Read the model definition and answer for the solid it produces. Units are mm, in the model's axes. Round coordinates to 2 decimals unless told otherwise and drop trailing zeros. Order: outer loops, then holes, each group sorted by start corner. A loop starts at its lowest first (then second) coordinate and runs counter-clockwise, first axis right, second up. Notation, with made-up numbers: (84.5, -8.75) - (90.5, -8.75) arc R26 cw to (90.5, 26.25) - close; hole circle Ø2 at (41.5, 60). An arc over 180 degrees is marked (long way). Answer as a JSON object with one key per item and string values. Group by question number.
Q1. Given pin 1 Ø2.5 at (y, z) = (-2, 1.5) entering from +X; pin 2 Ø1.5 at (x, y) = (-26, -2.5) entering from -Z; pin 3 Ø1 at (x, y) = (-6, -2.5) entering from -Z, each flat-ended and moving along its own axis, determine where each tip first touches the part or whether it passes through.
Q2. A cutting plane is placed at D-D on z = 83.5. Determine the outline of the cut face in (x, y), and give its area (3 significant figures).
Q3. A cutting plane is placed at C-C on y = -3.8. Count the separate pieces of the cut face and the enclosed holes in it, and give its area (3 significant figures).
Q4. A cutting plane is placed at A-A on z = -22. Determine the outline of the cut face in (x, y).
Q5. Consider line 1 (Z direction, x = 52.5, y = -4.3); line 2 (X direction, y = -3.75, z = 48); line 3 (X direction, y = -4, z = 62). Determine where each line is inside the solid, lowest interval first.
Q6. A cutting plane is placed at B-B on z = 108.5. Determine the outline of the cut face in (x, y), and give its area (3 significant figures).
```python
from build123d import *

# Parameters (mm, degrees)
SKETCH2_R           = 2.5
SKETCH2_W           = 5
SKETCH2_H           = 60
BOSS_EXTRUDE1_DEPTH = 5
BOSS_EXTRUDE2_DEPTH = 5


with BuildPart() as part:
    # Sketch2 → Boss-Extrude1 (new body)
    with BuildSketch(Plane(origin=(0, 0, 0), x_dir=(1, 0, 0), z_dir=(0, 1, 0))):
        with BuildLine():
            Line((45, 75), (75, 45))
            ThreePointArc((75, 45), (56.360389693, 0), (75, -45))
            Line((75, -45), (45, -75))
            ThreePointArc((45, -75), (0, -56.360389693), (-45, -75))
            Line((-45, -75), (-75, -45))
            ThreePointArc((-75, -45), (-56.360389693, 0), (-75, 45))
            Line((-75, 45), (-45, 75))
            ThreePointArc((-45, 75), (0, 56.360389693), (45, 75))
        make_face()
        with Locations(Location((50.841633347, 30.621504688, 0), (0, 0, 270))):
            Circle(SKETCH2_R, mode=Mode.SUBTRACT)
        with Locations(Location((61.448235065, 41.228106405, 0), (0, 0, 270))):
            Circle(SKETCH2_R, mode=Mode.SUBTRACT)
        with Locations(Location((30.621504688, 50.841633347, 0), (0, 0, 90))):
            Circle(SKETCH2_R, mode=Mode.SUBTRACT)
        with Locations(Location((41.228106405, 61.448235065, 0), (0, 0, 90))):
            Circle(SKETCH2_R, mode=Mode.SUBTRACT)
        with Locations(Location((30.621504688, -50.841633347, 0), (0, 0, 270))):
            Circle(SKETCH2_R, mode=Mode.SUBTRACT)
        with Locations(Location((41.228106405, -61.448235065, 0), (0, 0, 270))):
            Circle(SKETCH2_R, mode=Mode.SUBTRACT)
        with Locations(Location((61.448235065, -41.228106405, 0), (0, 0, 90))):
            Circle(SKETCH2_R, mode=Mode.SUBTRACT)
        with Locations(Location((50.841633347, -30.621504688, 0), (0, 0, 90))):
            Circle(SKETCH2_R, mode=Mode.SUBTRACT)
        with Locations(Location((-50.841633347, -30.621504688, 0), (0, 0, 270))):
            Circle(SKETCH2_R, mode=Mode.SUBTRACT)
        with Locations(Location((-61.448235065, -41.228106405, 0), (0, 0, 270))):
            Circle(SKETCH2_R, mode=Mode.SUBTRACT)
        with Locations(Location((-41.228106405, -61.448235065, 0), (0, 0, 90))):
            Circle(SKETCH2_R, mode=Mode.SUBTRACT)
        with Locations(Location((-30.621504688, -50.841633347, 0), (0, 0, 90))):
            Circle(SKETCH2_R, mode=Mode.SUBTRACT)
        with Locations(Location((-30.621504688, 50.841633347, 0), (0, 0, 270))):
            Circle(SKETCH2_R, mode=Mode.SUBTRACT)
        with Locations(Location((-41.228106405, 61.448235065, 0), (0, 0, 270))):
            Circle(SKETCH2_R, mode=Mode.SUBTRACT)
        with Locations(Location((-61.448235065, 41.228106405, 0), (0, 0, 90))):
            Circle(SKETCH2_R, mode=Mode.SUBTRACT)
        with Locations(Location((-50.841633347, 30.621504688, 0), (0, 0, 90))):
            Circle(SKETCH2_R, mode=Mode.SUBTRACT)
        with BuildLine():
            Line((38.610248674, 42.852889361), (42.852889361, 38.610248674))
            ThreePointArc((42.852889361, 38.610248674), (44.267102923, 38.024462236), (45.681316486, 38.610248674))
            Line((45.681316486, 38.610248674), (56.995024985, 49.923957173))
            ThreePointArc((56.995024985, 49.923957173), (57.580811422, 51.338170735), (56.995024985, 52.752384297))
            Line((56.995024985, 52.752384297), (52.752384297, 56.995024985))
            ThreePointArc((52.752384297, 56.995024985), (51.338170735, 57.580811422), (49.923957173, 56.995024985))
            Line((49.923957173, 56.995024985), (38.610248674, 45.681316486))
            ThreePointArc((38.610248674, 45.681316486), (38.024462236, 44.267102923), (38.610248674, 42.852889361))
        make_face(mode=Mode.SUBTRACT)
        with Locations((5, 0)):
            Rectangle(SKETCH2_W, SKETCH2_H, mode=Mode.SUBTRACT)
        with Locations((-5, 0)):
            Rectangle(SKETCH2_W, SKETCH2_H, mode=Mode.SUBTRACT)
        with BuildLine():
            Line((45.681316486, -38.610248674), (56.995024985, -49.923957173))
            ThreePointArc((56.995024985, -49.923957173), (57.580811422, -51.338170735), (56.995024985, -52.752384297))
            Line((56.995024985, -52.752384297), (52.752384297, -56.995024985))
            ThreePointArc((52.752384297, -56.995024985), (51.338170735, -57.580811422), (49.923957173, -56.995024985))
            Line((49.923957173, -56.995024985), (38.610248674, -45.681316486))
            ThreePointArc((38.610248674, -45.681316486), (38.024462236, -44.267102923), (38.610248674, -42.852889361))
            Line((38.610248674, -42.852889361), (42.852889361, -38.610248674))
            ThreePointArc((42.852889361, -38.610248674), (44.267102923, -38.024462236), (45.681316486, -38.610248674))
        make_face(mode=Mode.SUBTRACT)
        with BuildLine():
            Line((-38.610248674, -45.681316486), (-49.923957173, -56.995024985))
            ThreePointArc((-49.923957173, -56.995024985), (-51.338170735, -57.580811422), (-52.752384297, -56.995024985))
            Line((-52.752384297, -56.995024985), (-56.995024985, -52.752384297))
            ThreePointArc((-56.995024985, -52.752384297), (-57.580811422, -51.338170735), (-56.995024985, -49.923957173))
            Line((-56.995024985, -49.923957173), (-45.681316486, -38.610248674))
            ThreePointArc((-45.681316486, -38.610248674), (-44.267102923, -38.024462236), (-42.852889361, -38.610248674))
            Line((-42.852889361, -38.610248674), (-38.610248674, -42.852889361))
            ThreePointArc((-38.610248674, -42.852889361), (-38.024462236, -44.267102923), (-38.610248674, -45.681316486))
        make_face(mode=Mode.SUBTRACT)
        with BuildLine():
            Line((-45.681316486, 38.610248674), (-56.995024985, 49.923957173))
            ThreePointArc((-56.995024985, 49.923957173), (-57.580811422, 51.338170735), (-56.995024985, 52.752384297))
            Line((-56.995024985, 52.752384297), (-52.752384297, 56.995024985))
            ThreePointArc((-52.752384297, 56.995024985), (-51.338170735, 57.580811422), (-49.923957173, 56.995024985))
            Line((-49.923957173, 56.995024985), (-38.610248674, 45.681316486))
            ThreePointArc((-38.610248674, 45.681316486), (-38.024462236, 44.267102923), (-38.610248674, 42.852889361))
            Line((-38.610248674, 42.852889361), (-42.852889361, 38.610248674))
            ThreePointArc((-42.852889361, 38.610248674), (-44.267102923, 38.024462236), (-45.681316486, 38.610248674))
        make_face(mode=Mode.SUBTRACT)
        with Locations((-15, 0)):
            Rectangle(SKETCH2_W, SKETCH2_H, mode=Mode.SUBTRACT)
        with Locations((-25, 0)):
            Rectangle(SKETCH2_W, SKETCH2_H, mode=Mode.SUBTRACT)
        with Locations((15, 0)):
            Rectangle(SKETCH2_W, SKETCH2_H, mode=Mode.SUBTRACT)
        with Locations((25, 0)):
            Rectangle(SKETCH2_W, SKETCH2_H, mode=Mode.SUBTRACT)
    extrude(amount=-BOSS_EXTRUDE1_DEPTH)

    # Sketch3 → Boss-Extrude2 (add)
    with BuildSketch(Plane(origin=(0, 0, 0), x_dir=(1, 0, 0), z_dir=(0, 1, 0))):
        with BuildLine():
            Line((-20, -120), (20, -120))
            ThreePointArc((20, -120), (26.669664366, -94.260924648), (45, -75))
            ThreePointArc((45, -75), (0, -56.360389693), (-45, -75))
            ThreePointArc((-45, -75), (-26.669664366, -94.260924648), (-20, -120))
        make_face()
    extrude(amount=-BOSS_EXTRUDE2_DEPTH)


solid = part.part
```
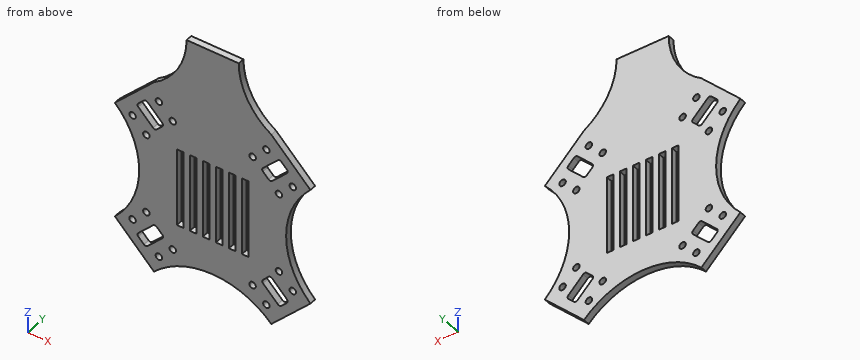
Result set:
{
 "1": {"pin 1": "stops at x = 56.42", "pin 2": "stops at z = -62.26", "pin 3": "stops at z = -56.69"},
 "2": {"outline": "(-34.57, -5) - (34.57, -5) - (34.57, 0) - (-34.57, 0) - close", "area": "346 mm²"},
 "3": {"separate pieces": "1", "enclosed holes": "26", "area": "16,800 mm²"},
 "4": {"outline": "(-60.28, -5) - (-27.5, -5) - (-27.5, 0) - (-60.28, 0) - close; (-22.5, -5) - (-17.5, -5) - (-17.5, 0) - (-22.5, 0) - close; (-12.5, -5) - (-7.5, -5) - (-7.5, 0) - (-12.5, 0) - close; (-2.5, -5) - (2.5, -5) - (2.5, 0) - (-2.5, 0) - close; (7.5, -5) - (12.5, -5) - (12.5, 0) - (7.5, 0) - close; (17.5, -5) - (22.5, -5) - (22.5, 0) - (17.5, 0) - close; (27.5, -5) - (60.28, -5) - (60.28, 0) - (27.5, 0) - close"},
 "5": {"line 1": "z = -67.5 to -57.21, -45.43 to -32.49, -28.75 to 28.75, 32.49 to 45.43, 57.21 to 67.5", "line 2": "x = -72 to -55.07, -40.93 to 40.93, 55.07 to 72", "line 3": "x = -58 to -43.67, -38.79 to 38.79, 43.67 to 58"},
 "6": {"outline": "(-21.26, -5) - (21.26, -5) - (21.26, 0) - (-21.26, 0) - close", "area": "213 mm²"}
}
